Input: dimensioned drawing with shaded views. Units: mm. Origin: part minimum x, y, z. A direction names the side the tool comes from. Coordinates: 2 decimals unless noted, no trailing zeros. Order: outer loops, then holes, each group sorted by start corner. A loop starts at its lowest first (then second) coordinate and runs counter-clockwise, first axis right, second up. Notation, with made-up numbers: (-32.75, 62) -> (-3.75, 62) arc R18 ccw to (-3.75, 81) -> close; hole circle Ø10 at (47, 87.25). An arc over 180 degrees is marked (long way). Answer as CSV lines item,"result".
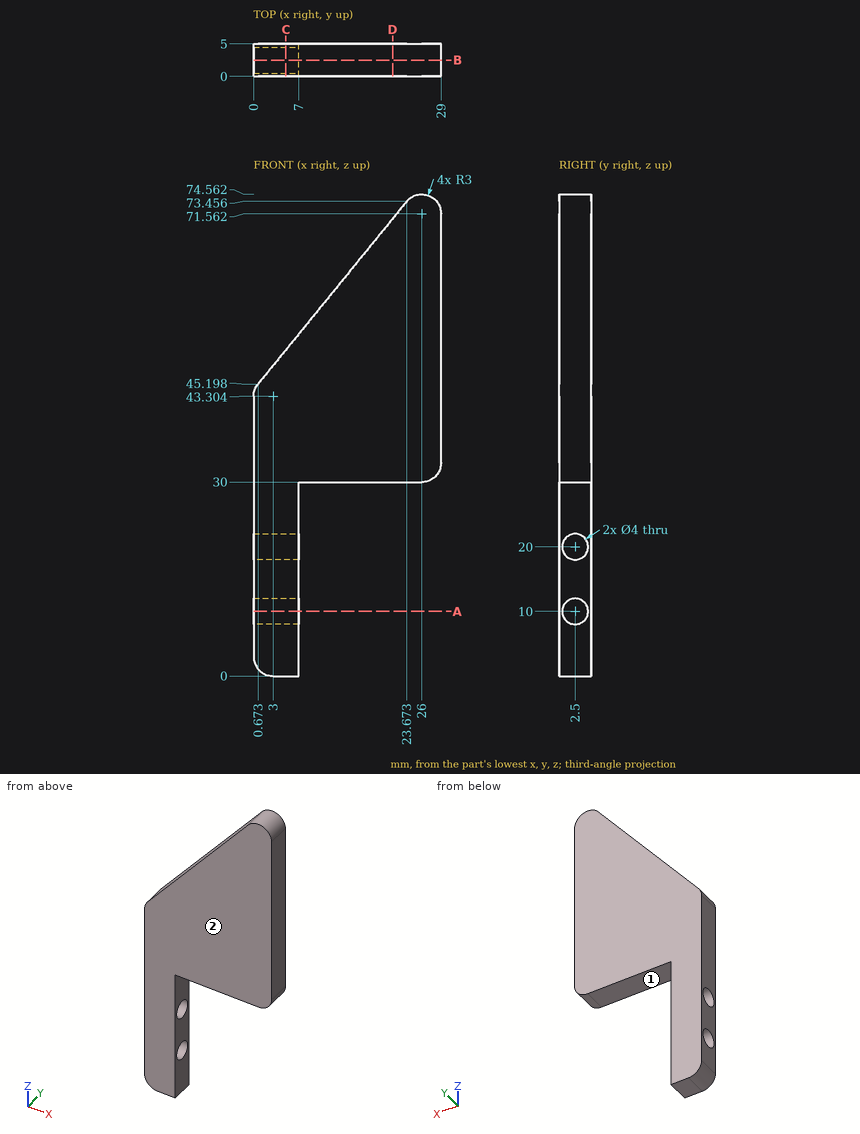
1. Cut plane A-A (z = 10). Return the cut outline in (x, y).
Findings:
outline,"(0, 0) -> (7, 0) -> (7, 0.5) -> (0, 0.5) -> close; (0, 4.5) -> (7, 4.5) -> (7, 5) -> (0, 5) -> close"
2. Cut plane C-C (x = 5). Return the cut outline in (y, z).
Findings:
outline,"(0, 0) -> (5, 0) -> (5, 50.51) -> (0, 50.51) -> close; hole circle Ø4 at (2.5, 10); hole circle Ø4 at (2.5, 20)"
3. Contact query for flat-ended pins moving along their axis: pin 1 (2 mm diameter, centred on x = 25, y = 0.5, fed in from -Z); pin 2 (1.5 mm diameter, centred on y = 0.5, z = 50, fed in from -X). Output: stop coordinate, or through.
Findings:
pin 1,"stops at z = 30"
pin 2,"stops at x = 3.97"
4. Reachability of the marked faces 1 and 2 from +Z, -Z, +X, -X, +Y, -Y: full face, straight path, thin tool, end or side. Return the list, or none.
Findings:
face 1,"-Z, +X, +Y, -Y"
face 2,"+Z, -Z, +X, -X, -Y"
5. Cut plane B-B (y = 2.5). Return the cut outline in (x, z) (1 decimal), plus the area to 3 significant figures.
Findings:
outline,"(0, 3) arc R3 ccw to (3, 0) -> (7, 0) -> (7, 8) -> (0, 8) -> close; (0, 12) -> (7, 12) -> (7, 18) -> (0, 18) -> close; (0, 22) -> (7, 22) -> (7, 30) -> (26, 30) arc R3 ccw to (29, 33) -> (29, 71.6) arc R3 ccw to (23.7, 73.5) -> (0.7, 45.2) arc R3 ccw to (0, 43.3) -> close"
area,"1,070 mm2"
6. Ray query, line 1 along Y through (x, z) = (3, 10); line 2 along Z through (x, y) = (2, 2.95); line 3 along X through (y, z) = (4.6, 4). Return the intervals inside material, ascending.
Findings:
line 1,"y = 0 to 0.5, 4.5 to 5"
line 2,"z = 0.17 to 8.05, 11.95 to 18.05, 21.95 to 46.83"
line 3,"x = 0 to 7"
7. Cut plane D-D (x = 21.5). Return the cut outline in (y, z) (1 decimal), plus the area to 3 significant figures.
Findings:
outline,"(0, 30) -> (5, 30) -> (5, 70.8) -> (0, 70.8) -> close"
area,"204 mm2"
